from build123d import *

# Parameters (mm, degrees)
SKETCH3_R               = 19.05
SKETCH3_R_2             = 14.351
CUT_EXTRUDE1_DEPTH      = 6.08
CUT_EXTRUDE1_DEPTH_BACK = 6.08


with BuildPart() as part:
    # Sketch1 → Revolve1 (revolve)
    with BuildSketch(Plane.XY):
        Polygon((-2.032, 0), (-3.175, 0), (-3.175, 2.794), (-5.08, 2.794), (-5.08, 4.318), (-2.032, 4.318), align=None)
    revolve(axis=Axis((0, 0, 0), (0, 1, 0)))

    # Sketch3 → Cut-Extrude1 (cut, two sides)
    with BuildSketch(Plane.XY) as cut_extrude1_sk:
        with Locations((0, -9.906)):
            Circle(SKETCH3_R)
        with Locations((0, -9.906)):
            Circle(SKETCH3_R_2, mode=Mode.SUBTRACT)
    extrude(amount=CUT_EXTRUDE1_DEPTH, mode=Mode.SUBTRACT)
    extrude(cut_extrude1_sk.sketch, amount=-CUT_EXTRUDE1_DEPTH_BACK, mode=Mode.SUBTRACT)


solid = part.part
CAD build for the part. Positions are in the model's coordinates, mm. A direction names the side the tool comes from. Coordinates: 2 decimals unless noted, no trailing zeros. Write each loop counter-clockwise with the first axis right and the second up, starting at its lowest first coordinate (ties: lowest second). Pieces come first, ordered by that corner, then holes. Notation, with made-up numbers: M 43.5,5 L 95.5,5 A26 cw 95.5,24 Z; hole C -28.75,-37 d2. An arc over 180 degrees is marked long. Answer as a JSON object with one key per item and string values. Group by question number.
1) Saw through at A-A (x = 0). Write the cut outline in (y, z) (3 decimals).
2) Pin check, flat tips, straight feed: pin 1 Ø2 at (x, y) = (-1.5, 3) entering from -Z; pin 2 Ø5 at (x, z) = (-1, -1.5) entering from +Y; pin 3 Ø2 at (y, z) = (3, 4) entering from +X; pin 4 Ø1.5 at (x, y) = (-3.5, 2) entering from +Z. Stop position of each tip, or through.
3) Saw through at D-D (z = 3). Write the cut outline in (x, y) (3 decimals), plus the area to 3 significant figures.
4) Tool access for faces 1 (the face through (3.3, 2.794, -1.1)), 2 (the face through (0, 4.318, -3)): list every direction of +Z, -Z, +X, -X, +Y, -Y with a clear straight run to the whole face (end or side of a thin tool).
5) Wall check: line 1 (Z direction, x = 0, y = 2.2) (3 decimals); line 2 (X direction, y = 2.9, z = 0); line 3 (Y direction, x = 1, z = 3.75). Give the ranges that are in metal, low to high. Write a range as from..to.
6) Saw through at C-C (z = 0). Write the cut outline in (x, y) (3 decimals), plus the area to 3 significant figures.
7) Saw through at B-B (y = 2.95). Write the cut outline in (x, z).
8) Mould opens along Z. For faces 3 (the face through (0.44, 2.129, -1.984)), 4 (the face through (0, 4.318, 3)), 5 (the face through (-4.69, 3.4, -1.95)) say: +Z half, -Z half, draft (parallel to the pull), parting line (faces both ways), or undercut.
Values follow:
{
 "1": {"outline": "M 0,-3.175 L 2.794,-3.175 L 2.794,-5.08 L 4.318,-5.08 L 4.318,-2.032 L 0,-2.032 Z; M 0,2.032 L 4.318,2.032 L 4.318,5.08 L 2.794,5.08 L 2.794,3.175 L 0,3.175 Z"},
 "2": {"pin 1": "stops at z = -5.06", "pin 2": "stops at y = 4.32", "pin 3": "stops at x = 4.1", "pin 4": "stops at z = 1.59"},
 "3": {"outline": "M -4.1,2.794 L -1.04,2.794 L -1.04,0 L 1.04,0 L 1.04,2.794 L 4.1,2.794 L 4.1,3.847 A14.351 ccw 1.905,4.318 L -1.905,4.318 A14.351 ccw -4.1,3.847 Z", "area": "17.4 mm2"},
 "4": {"face 1": "-Y", "face 2": "+Z, -Z, +X, -X, +Y"},
 "5": {"line 1": "z = -3.175..-2.032, 2.032..3.175", "line 2": "x = -5.08..-2.03, 2.03..5.08", "line 3": "y = 2.79..4.32"},
 "6": {"outline": "M -5.08,2.794 L -3.175,2.794 L -3.175,0 L -2.032,0 L -2.032,4.3 A14.351 ccw -5.08,3.516 Z; M 2.032,0 L 3.175,0 L 3.175,2.794 L 5.08,2.794 L 5.08,3.516 A14.351 ccw 2.032,4.3 Z", "area": "13.5 mm2"},
 "7": {"outline": "C 0,0 d10.16; hole C 0,0 d4.06"},
 "8": {"face 3": "undercut", "face 4": "draft", "face 5": "parting line"}
}
